from build123d import *

# Parameters (mm, degrees)
F0_W     = 3.81
F0_H     = 1.6002
F1_DEPTH = 13.0175
F0_W_2   = 11.6332
F0_H_2   = 0.9398
F2_DEPTH = 6.5913
F0_W_3   = 0.3048
F0_H_3   = 2.8448
F0_H_4   = 0.6604
F3_DEPTH = 7.1755
F0_H_5   = 2.54
F0_W_4   = 6.35
F0_H_6   = 1.4478
F4_DEPTH = 5.207
F0_W_5   = 5.08
F0_H_7   = 2.032
F5_DEPTH = 8.1788
F7_DEPTH = 3.6332


with BuildPart() as f1:
    # F0 (on Right) → F1 (new body, symmetric)
    with BuildSketch(Plane.YZ):
        Polygon((11.6332, 0), (0, 0), (0, -1.6002), (5.08, -1.6002), (10.16, -1.6002), (16.4592, -1.6002), (16.4592, 0), align=None)
        with Locations((18.3642, -0.8001)):
            Rectangle(F0_W, F0_H)
    extrude(amount=F1_DEPTH, both=True)

    # F0 (on Right) → F2 (join, symmetric)
    with BuildSketch(Plane.YZ):
        with Locations((5.8166, 0.4699)):
            Rectangle(F0_W_2, F0_H_2)
        Polygon((-2.5908, 0.9398), (0, 0.9398), (11.6332, 0.9398), (11.6332, 6.6294), (-2.5908, 6.6294), (-2.5908, 3.7846), align=None)
    extrude(amount=F2_DEPTH, both=True)

    # F0 (on Right) → F3 (join, symmetric)
    with BuildSketch(Plane.YZ):
        with Locations((-2.7432, 5.207)):
            Rectangle(F0_W_3, F0_H_3)
        with Locations((-2.7432, 6.9596)):
            Rectangle(F0_W_3, F0_H_4)
        with Locations((-2.7432, 2.3622)):
            Rectangle(F0_W_3, F0_H_3)
        with Locations((-2.7432, 0.6096)):
            Rectangle(F0_W_3, F0_H_4)
    extrude(amount=F3_DEPTH, both=True)

    # F0 (on Right) → F4 (join, symmetric)
    with BuildSketch(Plane.YZ):
        with Locations((18.3642, 1.27)):
            Rectangle(F0_W, F0_H_5)
        with Locations((23.4442, 1.27)):
            Rectangle(F0_W_4, F0_H_5)
        with Locations((18.3642, -2.3241)):
            Rectangle(F0_W, F0_H_6)
    extrude(amount=F4_DEPTH, both=True)

    # F0 (on Right) → F5 (join, symmetric)
    with BuildSketch(Plane.YZ):
        with Locations((7.62, -2.6162)):
            Rectangle(F0_W_5, F0_H_7)
    extrude(amount=F5_DEPTH, both=True)

    # F6 (on face) → F7 (cut, through all)
    with BuildSketch(Plane.XY):
        with BuildLine():
            Line((-10.4394, 4.2672), (-10.4394, 0.889))
            ThreePointArc((-10.4394, 0.889), (-9.245026, 1.383726), (-8.7503, 2.5781))
            ThreePointArc((-8.7503, 2.5781), (-9.245026, 3.772474), (-10.4394, 4.2672))
        make_face()
        with BuildLine():
            ThreePointArc((-12.1285, 2.5781), (-11.633774, 1.383726), (-10.4394, 0.889))
            Line((-10.4394, 0.889), (-10.4394, 4.2672))
            ThreePointArc((-10.4394, 4.2672), (-11.633774, 3.772474), (-12.1285, 2.5781))
        make_face()
        with BuildLine():
            Line((-10.4394, 19.3802), (-10.4394, 16.002))
            ThreePointArc((-10.4394, 16.002), (-9.245026, 16.496726), (-8.7503, 17.6911))
            ThreePointArc((-8.7503, 17.6911), (-9.245026, 18.885474), (-10.4394, 19.3802))
        make_face()
        with BuildLine():
            ThreePointArc((-12.1285, 17.6911), (-11.633774, 16.496726), (-10.4394, 16.002))
            Line((-10.4394, 16.002), (-10.4394, 19.3802))
            ThreePointArc((-10.4394, 19.3802), (-11.633774, 18.885474), (-12.1285, 17.6911))
        make_face()
        with BuildLine():
            ThreePointArc((8.7503, 17.6911), (9.245026, 16.496726), (10.4394, 16.002))
            Line((10.4394, 16.002), (10.4394, 19.3802))
            ThreePointArc((10.4394, 19.3802), (9.245026, 18.885474), (8.7503, 17.6911))
        make_face()
        with BuildLine():
            Line((10.4394, 19.3802), (10.4394, 16.002))
            ThreePointArc((10.4394, 16.002), (11.633774, 16.496726), (12.1285, 17.6911))
            ThreePointArc((12.1285, 17.6911), (11.633774, 18.885474), (10.4394, 19.3802))
        make_face()
        with BuildLine():
            ThreePointArc((8.7503, 2.5781), (9.245026, 1.383726), (10.4394, 0.889))
            Line((10.4394, 0.889), (10.4394, 4.2672))
            ThreePointArc((10.4394, 4.2672), (9.245026, 3.772474), (8.7503, 2.5781))
        make_face()
        with BuildLine():
            Line((10.4394, 4.2672), (10.4394, 0.889))
            ThreePointArc((10.4394, 0.889), (11.633774, 1.383726), (12.1285, 2.5781))
            ThreePointArc((12.1285, 2.5781), (11.633774, 3.772474), (10.4394, 4.2672))
        make_face()
    extrude(amount=-F7_DEPTH, mode=Mode.SUBTRACT)


solid = f1.part
Geometry: final body of the model. Coordinates: model frame, mm. A direction names the side the tool comes from. Round coordinates to 2 decimals unless told otherwise and drop trailing zeros. Loops run counter-clockwise (first coordinate to the right, second up) from the corner with the lowest first, then second, coordinate; pieces in that order, holes last. Notation, with made-up numbers: (-36, 64) - (1, 64) arc R9 cw to (1, 76) - close; hole circle Ø7 at (83.25, 41). An arc over 180 degrees is marked (long way). Write each question's results on one line, items separated by ' | '. Start each with the question number.
1) Cut plane B-B on y = 11. Return loops of the section in (x, z), then the cut area to 3 significant figures.
2) Cut plane D-D on y = 1.75. Return loops of the section in (x, z).
3) First-contact query: P1, Ø3, axis at x = 2.5, y = 18.5, coming from the -Z side; P2, Ø5, axis at x = 0, y = 24.5, coming from the -Z side; P3, Ø8, axis at x = -4, y = 11, coming from the +Z side. Flat tips, straight axial feed; report the tip coordinate or a pass-through.
4) Mould query, pull axis Y, two halves, no side actions, for faces 1 (the face through (8.179, 8, -3)), 2 (the face through (0, -1, 0.94)), 3 (the face through (0, 5.08, -3)). Classes: released by +Y, released by -Y, zero draft, split by the parting line, or undercut.
5) Cut plane A-A on z = 2. Return loops of the section in (x, y).
6) Access query for faces 4 (the face through (5.207, 18, -2)), 5 (the face through (-5.207, 18, -2)), 6 (the face through (0, 11.633, 3)), 7 (the face through (6.591, 4, 3)). Directions: +Z, -Z, +X, -X, +Y, -Y. A direction counts if a zero-diameter tool reaches every point of the face in a straight line with its end or side. Return the directions, or none.
7) Line query: probe 1 along Y at (x, z) = (0.5, -2); probe 2 along Z at (x, y) = (3.5, 2.75); probe 3 along Z at (x, y) = (-10.75, 11.75). Output: solid intervals per line, ascending. Write a range as [from, to].
8) Cut plane C-C on x = -3. Return loops of the section in (y, z), then the cut area to 3 significant figures.
Verdict:
1) outline: (-13.02, -1.6) - (13.02, -1.6) - (13.02, 0) - (6.59, 0) - (6.59, 6.63) - (-6.59, 6.63) - (-6.59, 0) - (-13.02, 0) - close | area: 129 mm2
2) outline: (-13.02, -1.6) - (-11.91, -1.6) - (-11.91, 0) - (-13.02, 0) - close; (-8.97, -1.6) - (8.97, -1.6) - (8.97, 0) - (6.59, 0) - (6.59, 6.63) - (-6.59, 6.63) - (-6.59, 0) - (-8.97, 0) - close; (11.91, -1.6) - (13.02, -1.6) - (13.02, 0) - (11.91, 0) - close
3) P1: stops at z = -3.05 | P2: stops at z = 0 | P3: stops at z = 6.63
4) face 1: zero draft | face 2: undercut | face 3: released by -Y
5) outline: (-7.18, -2.9) - (7.18, -2.9) - (7.18, -2.59) - (6.59, -2.59) - (6.59, 11.63) - (-6.59, 11.63) - (-6.59, -2.59) - (-7.18, -2.59) - close; (-5.21, 16.46) - (5.21, 16.46) - (5.21, 26.62) - (-5.21, 26.62) - close
6) face 4: -Z, +X, +Y | face 5: -Z, -X, +Y | face 6: +Z, +X, -X | face 7: +Z, +X, +Y
7) probe 1: y = [5.08, 10.16], [16.46, 20.27] | probe 2: z = [-1.6, 6.63] | probe 3: z = [-1.6, 0]
8) outline: (-2.9, 0.28) - (-2.59, 0.28) - (-2.59, 0.94) - (0, 0.94) - (0, -1.6) - (5.08, -1.6) - (5.08, -3.63) - (10.16, -3.63) - (10.16, -1.6) - (16.46, -1.6) - (16.46, -3.05) - (20.27, -3.05) - (20.27, 0) - (26.62, 0) - (26.62, 2.54) - (16.46, 2.54) - (16.46, 0) - (11.63, 0) - (11.63, 6.63) - (-2.59, 6.63) - (-2.59, 7.29) - (-2.9, 7.29) - close | area: 168 mm2
